Verification items for this drawing (mm, ordinates from the low corner). A direction names the side the tool comes from. Give positions to 0.01 mm unless a question says otherwise; leave off trailing zeros. Write each loop counter-clockwise with the first axis right and the second up, starting at its lowest first coordinate (ties: lowest second). Pieces come first, ordered by that corner, then holes. Notation, with made-up numbers: (-26, 38.5) -> (-18, 38.5) arc R16 ccw to (-18, 63.5) -> close; hole circle Ø5 at (89, 83). An arc over 180 degrees is marked (long way). One line per item, written item: value.
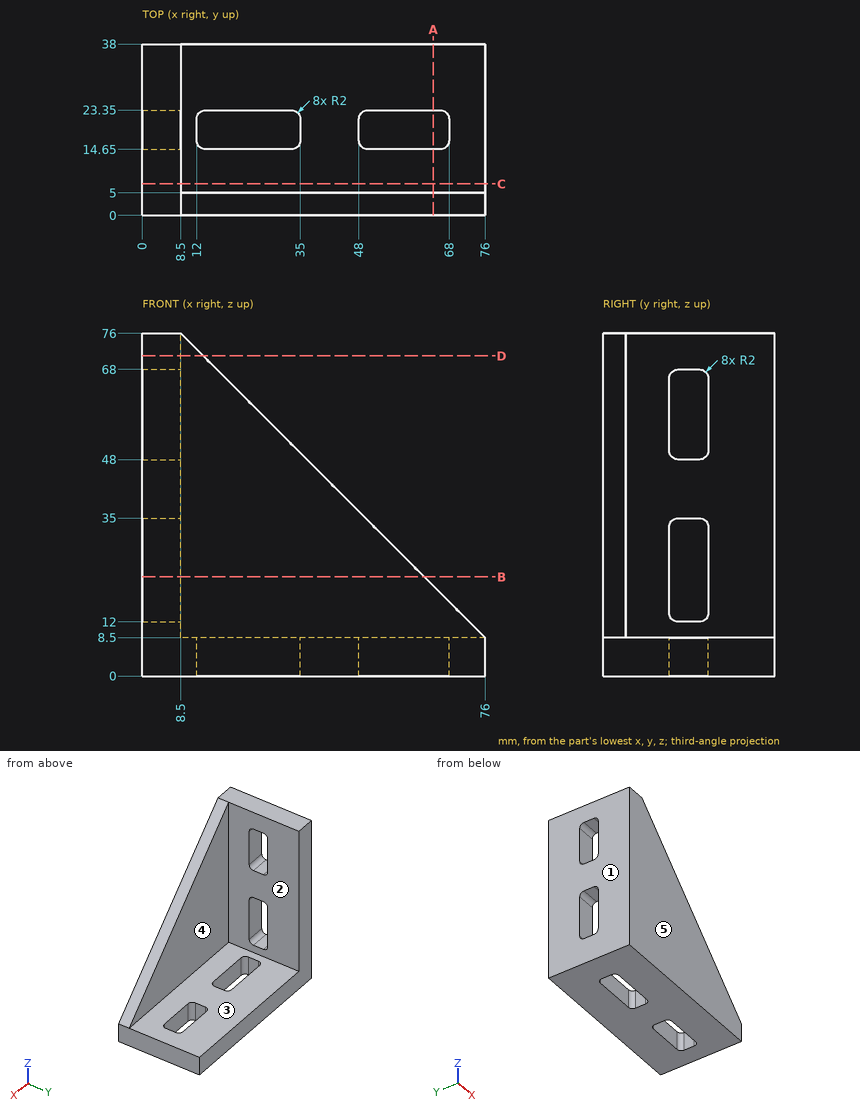
1) Sectioned sample at C-C on y = 7. Record the cut outline in (x, z).
Verdict:
outline: (0, 0) -> (76, 0) -> (76, 8.5) -> (8.5, 8.5) -> (8.5, 76) -> (0, 76) -> close
2) Depth check by flat-ended pin: pin 1 Ø1.5 at (x, y) = (57.5, 11.5) entering from +Z; pin 2 Ø10 at (y, z) = (13, 41.5) entering from +X; pin 3 Ø1 at (x, z) = (38.5, 34.5) entering from +Y; pin 4 Ø1.5 at (x, y) = (32.5, 19.5) entering from +Z. Enter the tip coordinate at first touch or a pass-through.
Verdict:
pin 1: z = 8.5
pin 2: x = 8.5
pin 3: y = 5
pin 4: through
3) Mould release check, pull along Y, two halves, no side actions. Record for the marked faces 3, 4 and 5: released by +Y, released by -Y, zero draft, split by the parting line, or undercut.
Verdict:
face 3: zero draft
face 4: released by +Y
face 5: released by -Y
4) Tool access check on the marked faces 1 and 2. Record the directions out of +Z, -Z, +X, -X, +Y, -Y that give a thin tool (end or side, any length) a straight path to the whole face; none if there is none.
Verdict:
face 1: +Z, -Z, -X, +Y, -Y
face 2: +Z, +X, +Y
5) Sectioned sample at B-B on z = 22. Record the cut outline in (x, y).
Verdict:
outline: (0, 0) -> (62.5, 0) -> (62.5, 5) -> (8.5, 5) -> (8.5, 14.65) -> (0, 14.65) -> close; (0, 23.35) -> (8.5, 23.35) -> (8.5, 38) -> (0, 38) -> close
6) Scan lines: probe 1 along Y at (x, z) = (47.5, 30.5); probe 2 along X at (y, z) = (23.5, 32). Record each from-to range of solid material in increasing order.
Verdict:
probe 1: 0 to 5
probe 2: 0 to 8.5
7) Sectioned sample at A-A on x = 64.5. Record the cut outline in (y, z), plus the area to 3 significant figures.
Verdict:
outline: (0, 0) -> (14.65, 0) -> (14.65, 8.5) -> (5, 8.5) -> (5, 20) -> (0, 20) -> close; (23.35, 0) -> (38, 0) -> (38, 8.5) -> (23.35, 8.5) -> close
area: 307 mm^2
8) Sectioned sample at D-D on z = 71. Record the cut outline in (x, y).
Verdict:
outline: (0, 0) -> (13.5, 0) -> (13.5, 5) -> (8.5, 5) -> (8.5, 38) -> (0, 38) -> close
